The drawing under review shows one solid part. Ordinate dimensions are in mm from its lowest x, y, z. A direction names the side the tool comes from. Coordinates: 2 decimals unless noted, no trailing zeros. Write each loop counter-clockwise with the first axis right and the second up, starting at its lowest first coordinate (ties: lowest second). Pieces come first, ordered by that corner, then holes. Notation, with made-up numbers: (-36.75, 43.5) - (-4.75, 43.5) arc R10 cw to (-4.75, 59.5) - close; hole circle Ø8 at (-36.75, 45.25). An arc over 180 degrees is marked (long way). Use a Markdown table: item, result.
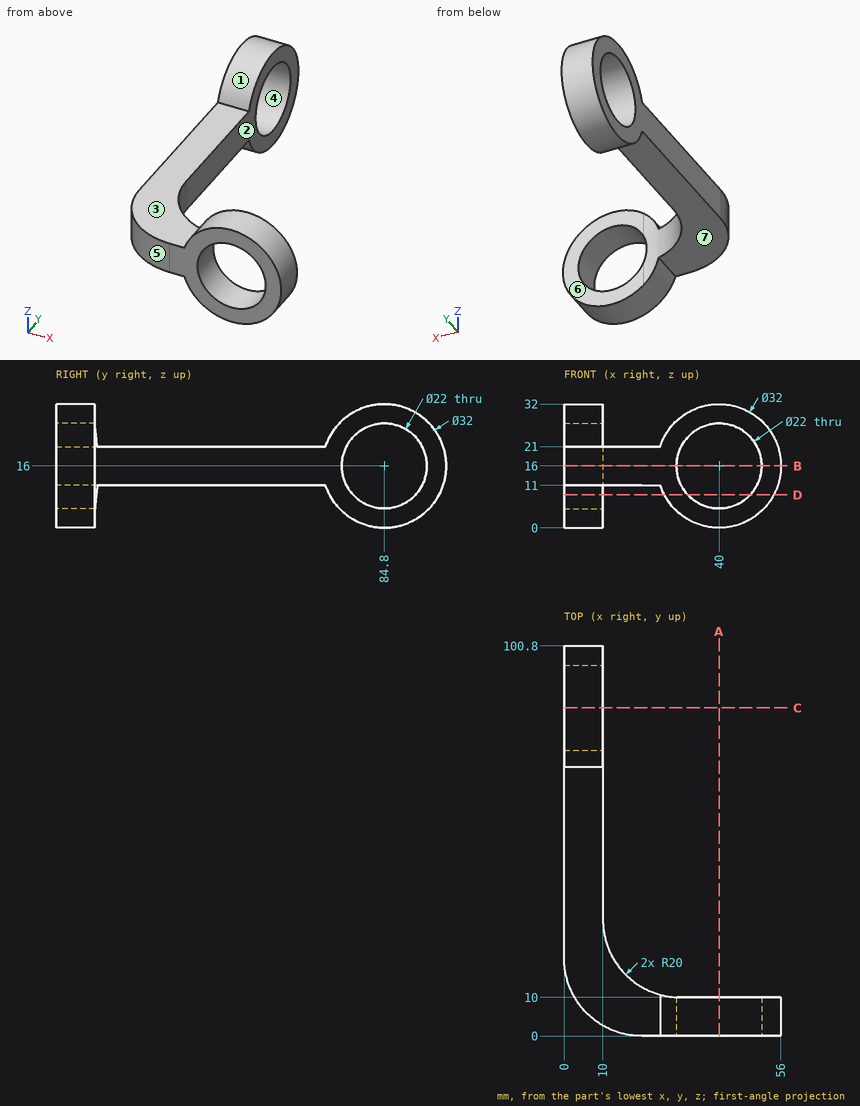
(1) Take a section at B-B on z = 16. Write out the cut boundary in (x, y), and give its area (3 significant figures).
Determined:
| item | result |
|---|---|
| outline | (0, 20) arc R20 ccw to (20, 0) - (29, 0) - (29, 10.03) arc R20 cw to (10, 30) - (10, 73.8) - (0, 73.8) - close; (0, 95.8) - (10, 95.8) - (10, 100.8) - (0, 100.8) - close; (51, 0) - (56, 0) - (56, 10) - (51, 10) - close |
| area | 1,030 mm2 |
(2) For L1, parallel to Z at x = 3, y = 84.8; L2, parallel to Z at x = 7.5, y = 23.5; L3, parallel to Y at x = 46, z = 6, list the stretches that pass through material, from the lowest coordinate up. Write a range as from..to.
Determined:
| item | result |
|---|---|
| L1 | 0..5, 27..32 |
| L2 | 11..21 |
| L3 | 0..10 |
(3) For pin 1 (16 mm diameter, centred on y = 58.5, z = 14, fed in from +X); pin 2 (13 mm diameter, centred on x = 49, z = 23.5, fed in from +Y); pin 3 (20 mm diameter, centred on x = 9, y = 24, fed in from +Z), all flat-tipped, find the tip position at first contact; note any pin that passes through.
Determined:
| item | result |
|---|---|
| pin 1 | x = 10 |
| pin 2 | y = 10 |
| pin 3 | z = 21 |
(4) Draft analysis for pull direction Y (two halves, no side actions). For the marked faces 4, 5, 6 and 7, state which applies: +Y half, -Y half, draft (parallel to the pull), parting line (faces both ways), or undercut.
Determined:
| item | result |
|---|---|
| face 4 | undercut |
| face 5 | -Y half |
| face 6 | +Y half |
| face 7 | draft |
(5) Machinability: for the marked faces 1, 2 and 3, which of the approach directions +Z, -Z, +X, -X, +Y, -Y give a long, thin tool a straight path to every point of the face, cutting with its end or side? Answer none if there is none.
Determined:
| item | result |
|---|---|
| face 1 | +X, -X |
| face 2 | +Z, -Z, +X, +Y |
| face 3 | +Z, -X, -Y |
(6) Take a section at D-D on z = 8.5. Write out the cut boundary in (x, y).
Determined:
| item | result |
|---|---|
| outline | (0, 70.67) - (10, 70.67) - (10, 76.75) - (0, 76.75) - close; (0, 92.85) - (10, 92.85) - (10, 98.93) - (0, 98.93) - close; (25.87, 0) - (31.95, 0) - (31.95, 10) - (30, 10) arc R20 cw to (25.87, 10.43) - close; (48.05, 0) - (54.13, 0) - (54.13, 10) - (48.05, 10) - close |
(7) Take a section at A-A on x = 40. Write out the cut boundary in (y, z).
Determined:
| item | result |
|---|---|
| outline | (0, 0) - (10, 0) - (10, 5) - (0, 5) - close; (0, 27) - (10, 27) - (10, 32) - (0, 32) - close |
